from build123d import *


with BuildPart() as f1:
    # F0 (on Front) → F1 (revolve)
    with BuildSketch(Plane.XZ):
        Polygon((1.3, 14.5), (1.573288, 1.2), (2.4, 1.2), (2.4, 3.7), (2, 5.7), (2.4, 6.2), (2.310274, 6.7), (2.160274, 6.7), (2, 14.5), align=None)
        Polygon((0, 1.2), (0, 0), (5, 0), (5, 1.2), (2.4, 1.2), (1.573288, 1.2), align=None)
    revolve(axis=Axis((0, 0, 7.25), (0, 0, 1)))


solid = f1.part
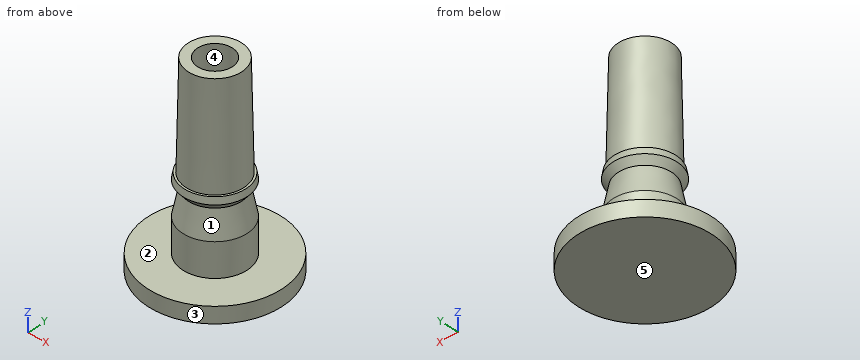
Verification items for the finished model (mm, model axes). Face numbers are marked on the shaded views. A direction names the side the tool comes from. Coordinates: 2 decimals unless noted, no trailing zeros. Order: outer loops, then holes, each group sorted by start corner. A loop starts at its lowest first (then second) coordinate and runs counter-clockwise, first axis right, second up. Notation, with made-up numbers: (11.25, 87) -> (48.25, 87) arc R17 ccw to (48.25, 103) -> close; hole circle Ø4 at (5, 78). An arc over 180 degrees is marked (long way). Use CSV: the item, a comma, the result in double quotes. Start each with the question number.
Q1. Thickness scan on line 1 along Z through (x, y) = (4, -2.5); line 2 along Y through (x, z) = (-0.25, 12.75); line 3 along X through (y, z) = (0, 10.5). Record the ranges inside material, lowest first.
Q2. Depth check by flat-ended pin: P1, Ø5, axis at y = -2, z = 4, coming from the +X side; P2, Ø3, axis at y = -0.5, z = 11.5, coming from the +X side. Enter the tip coordinate at first touch or a pass-through.
Q3. Section check A-A, the plane x = 0. Record the cut outline in (y, z), and give its area (3 significant figures).
Q4. Section check C-C, the plane z = 8. Record the cut outline in (x, y), and give its area (3 significant figures).
Q5. Tool access check on the marked faces 1 and 2. Record the directions out of +Z, -Z, +X, -X, +Y, -Y that give a thin tool (end or side, any length) a straight path to the whole face; none if there is none.
Q6. Section check D-D, the plane x = -4. Record the cut outline in (y, z).
Q7. Draft check along X on the marked faces 3, 4 and 5. Enter one of: +X half, -X half, draft (parallel to the pull), parting line (faces both ways), or undercut.
Returned:
1,line 1,"z = 0 to 1.2"
1,line 2,"y = -2.02 to -1.31, 1.31 to 2.02"
1,line 3,"x = -2.08 to -1.38, 1.38 to 2.08"
2,P1,"stops at x = 2.4"
2,P2,"stops at x = 2.09"
3,outline,"(-5, 0) -> (5, 0) -> (5, 1.2) -> (2.4, 1.2) -> (2.4, 3.7) -> (2, 5.7) -> (2.4, 6.2) -> (2.31, 6.7) -> (2.16, 6.7) -> (2, 14.5) -> (1.3, 14.5) -> (1.57, 1.2) -> (-1.57, 1.2) -> (-1.3, 14.5) -> (-2, 14.5) -> (-2.16, 6.7) -> (-2.31, 6.7) -> (-2.4, 6.2) -> (-2, 5.7) -> (-2.4, 3.7) -> (-2.4, 1.2) -> (-5, 1.2) -> close"
3,area,"31.6 mm^2"
4,outline,"circle Ø4.27 at (0, 0); hole circle Ø2.87 at (0, 0)"
4,area,"7.84 mm^2"
5,face 1,"none"
5,face 2,"+Z"
6,outline,"(-3, 0) -> (3, 0) -> (3, 1.2) -> (-3, 1.2) -> close"
7,face 3,"parting line"
7,face 4,"undercut"
7,face 5,"draft"
